from build123d import *

# Parameters (mm, degrees)
SKETCH1_W           = 95
SKETCH1_H           = 20
SKETCH1_R           = 1.65
BOSS_EXTRUDE1_DEPTH = 4
SKETCH2_R           = 5.65
SKETCH2_R_2         = 1.65
EXTRUDE_THIN1_DEPTH = 2
CHAMFER1_SIZE       = 2
SKETCH3_R           = 7.65
SKETCH3_R_2         = 1.65
EXTRUDE_THIN2_DEPTH = 4
CHAMFER2_SIZE       = 4


with BuildPart() as part:
    # Sketch1 → Boss-Extrude1 (new body)
    with BuildSketch(Plane.XY):
        Rectangle(SKETCH1_W, SKETCH1_H)
        Circle(SKETCH1_R, mode=Mode.SUBTRACT)
        with Locations((25.5, 0)):
            Circle(SKETCH1_R, mode=Mode.SUBTRACT)
        with Locations((-25.5, 0)):
            Circle(SKETCH1_R, mode=Mode.SUBTRACT)
    extrude(amount=BOSS_EXTRUDE1_DEPTH)

    # Sketch2 → Extrude-Thin1 (add)
    # profile 1 of 2: a face of its own
    with BuildSketch(Plane.XY.offset(4)):
        with Locations((-25.5, 0)):
            Circle(SKETCH2_R)
        with Locations((-25.5, 0)):
            Circle(SKETCH2_R_2, mode=Mode.SUBTRACT)
    # profile 2 of 2: a face of its own
    with BuildSketch(Plane.XY.offset(4)):
        with Locations((25.5, 0)):
            Circle(SKETCH2_R)
        with Locations((25.5, 0)):
            Circle(SKETCH2_R_2, mode=Mode.SUBTRACT)
    extrude(amount=EXTRUDE_THIN1_DEPTH)

    # Chamfer1
    chamfer1_edges = [part.edges().sort_by_distance(p)[0] for p in [
        (-31.15, 0, 6),
        (19.85, 0, 6),
    ]]
    chamfer(chamfer1_edges, length=CHAMFER1_SIZE - 0.0001)  # a hair under: the kernel refuses the full size

    # Sketch3 → Extrude-Thin2 (add)
    with BuildSketch(Plane.XY.offset(4)):
        Circle(SKETCH3_R)
        Circle(SKETCH3_R_2, mode=Mode.SUBTRACT)
    extrude(amount=EXTRUDE_THIN2_DEPTH)

    # Chamfer2
    chamfer2_edges = [part.edges().sort_by_distance(p)[0] for p in [
        (-7.65, 0, 8),
    ]]
    chamfer(chamfer2_edges, length=CHAMFER2_SIZE - 0.0001)  # a hair under: the kernel refuses the full size


solid = part.part
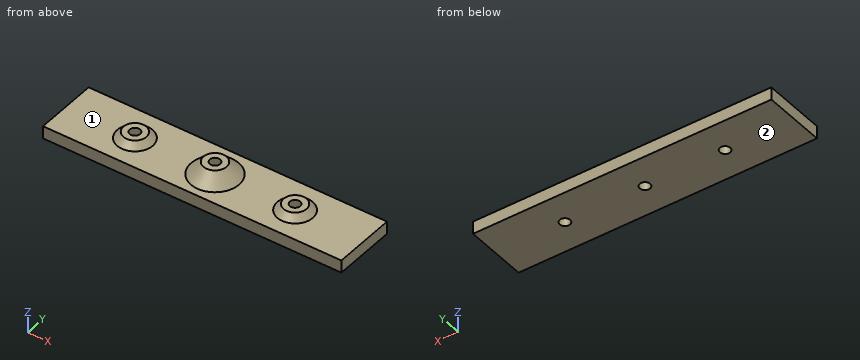
Check sheet for the modelled part. Datum: model origin and axes. Units: mm. Face numbers are marked on the shaded views. A direction names the side the tool comes from. Round coordinates to 2 decimals unless told otherwise and drop trailing zeros. Write each loop counter-clockwise with the first axis right and the second up, starting at its lowest first coordinate (ties: lowest second). Pieces come first, ordered by that corner, then holes. Notation, with made-up numbers: (51, 71.5) -> (61, 71.5) arc R32 cw to (61, 97.5) -> close; hole circle Ø7 at (-22, -21). An arc over 180 degrees is marked (long way). Answer as CSV lines item,"result". Start each with the question number.
1) Go/stop test with flat-tipped pins: P1, Ø3, axis at x = 25.5, y = 0, coming from the +Z side; P2, Ø2, axis at x = 24, y = -1, coming from the +Z side; P3, Ø10, axis at x = 12.5, y = 3.5, coming from the +Z side. Record where each tip stops, or that it passes through.
2) Section check A-A on y = 0. State how many separate pieces and enclosed holes the cut face has, and give its area (3 significant figures).
3) Tool access check on the marked faces 1 and 2. Record the directions out of +Z, -Z, +X, -X, +Y, -Y that give a thin tool (end or side, any length) a straight path to the whole face; none if there is none.
4) Material ranges on line 1 (Y direction, x = -25.5, z = 3.1); line 2 (Z direction, x = 6.5, y = 7.5); line 3 (X direction, y = 3.25, z = 5.25), recorded low to high. Write a range as from..to.
5) Section check D-D on x = -11.5. Enter the section's corners in (y, z).
Found:
1,P1,"passes through"
1,P2,"stops at z = 6"
1,P3,"stops at z = 4"
2,separate pieces,"4"
2,enclosed holes,"0"
2,area,"396 mm^2"
3,face 1,"+Z"
3,face 2,"-Z, +X, -X, +Y, -Y"
4,line 1,"y = -10..-1.65, 1.65..10"
4,line 2,"z = 0..4"
4,line 3,"x = -28.47..-22.53, -5.51..5.51, 22.53..28.47"
5,outline,"(-10, 0) -> (10, 0) -> (10, 4) -> (-10, 4) -> close"
